Part model, mm, in its own coordinate system. Face numbers are marked on the shaded views. A direction names the side the tool comes from. Coordinates: 2 decimals unless noted, no trailing zeros. Order: outer loops, then holes, each group sorted by start corner. A loop starts at its lowest first (then second) coordinate and runs counter-clockwise, first axis right, second up. Notation, with made-up numbers: M -13,87 L 6,87 A28 ccw 6,120 Z; hole C 76,7 d5. An arc over 180 degrees is marked long. Answer in a Markdown table with one row per item. Add a question column.
from build123d import *

# Parameters (mm, degrees)
F0_W     = 70
F0_H     = 100
F1_DEPTH = 50
F2_W     = 70
F2_H     = 50
F3_DEPTH = 25
F4_W     = 30
F4_H     = 50
F5_DEPTH = 15


with BuildPart() as f1:
    # F0 (on Top) → F1 (new body)
    with BuildSketch(Plane.XY):
        Rectangle(F0_W, F0_H)
    extrude(amount=F1_DEPTH)

    # F2 (on face) → F3 (cut)
    with BuildSketch(Plane.XY.offset(50)):
        with Locations((0, -25)):
            Rectangle(F2_W, F2_H)
    extrude(amount=-F3_DEPTH, mode=Mode.SUBTRACT)

    # F4 (on face) → F5 (cut)
    with BuildSketch(Plane.XY.offset(50)):
        with Locations((20, 25)):
            Rectangle(F4_W, F4_H)
    extrude(amount=-F5_DEPTH, mode=Mode.SUBTRACT)


solid = f1.part
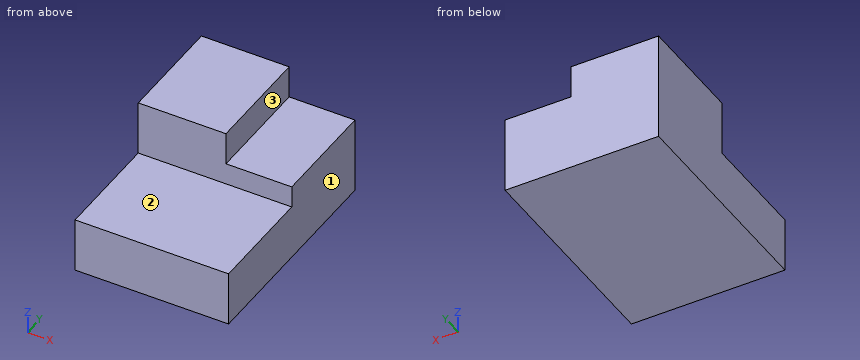
(1) Slice it at A-A (y = 36.5). List the corners of the cut face in (x, z), and give its area (3 significant figures).
(2) Wall check: line 1 (Y direction, x = 32, z = 31); line 2 (Z direction, x = 0, y = -12.5); line 3 (Z direction, x = 22.5, y = 28). Give the ranges that are in metal, low to high.
(3) Drop flat-ended pins along their axis: P1, Ø15, axis at x = 3, y = -22, coming from the +Z side; P2, Ø3, axis at x = -20.5, z = 37, coming from the -Y side; P3, Ø7.5, axis at y = 31.5, z = 42.5, coming from the +X side. Give the stop position or say it passes through.
(4) Slice it at B-B (x = -5.5). List the corners of the cut face in (y, z), and give its area (3 significant figures).
(5) 3-axis set-ups, long thin cutter, end or side, ignore diameter. For the marked faces 1, 2 and 3: which of +Z, -Z, +X, -X, +Y, -Y reach the whole face in a straight line?
(6) Slice it at D-D (z = 33.5). List the corners of the cut face in (x, y), and give its area (3 significant figures).
(7) Slice it at C-C (z = 43). List the corners of the cut face in (x, y).
Computed:
| question | item | result |
|---|---|---|
| 1 | outline | M -35,0 L 35,0 L 35,35 L 5,35 L 5,50 L -35,50 Z |
| 1 | area | 3,050 mm^2 |
| 2 | line 1 | y = 0 to 50 |
| 2 | line 2 | z = 0 to 25 |
| 2 | line 3 | z = 0 to 35 |
| 3 | P1 | stops at z = 25 |
| 3 | P2 | stops at y = 0 |
| 3 | P3 | stops at x = 5 |
| 4 | outline | M -50,0 L 50,0 L 50,50 L 0,50 L 0,25 L -50,25 Z |
| 4 | area | 3,750 mm^2 |
| 5 | face 1 | +Z, -Z, +X, +Y, -Y |
| 5 | face 2 | +Z, +X, -X, -Y |
| 5 | face 3 | +Z, +X, +Y, -Y |
| 6 | outline | M -35,0 L 35,0 L 35,50 L -35,50 Z |
| 6 | area | 3,500 mm^2 |
| 7 | outline | M -35,0 L 5,0 L 5,50 L -35,50 Z |
